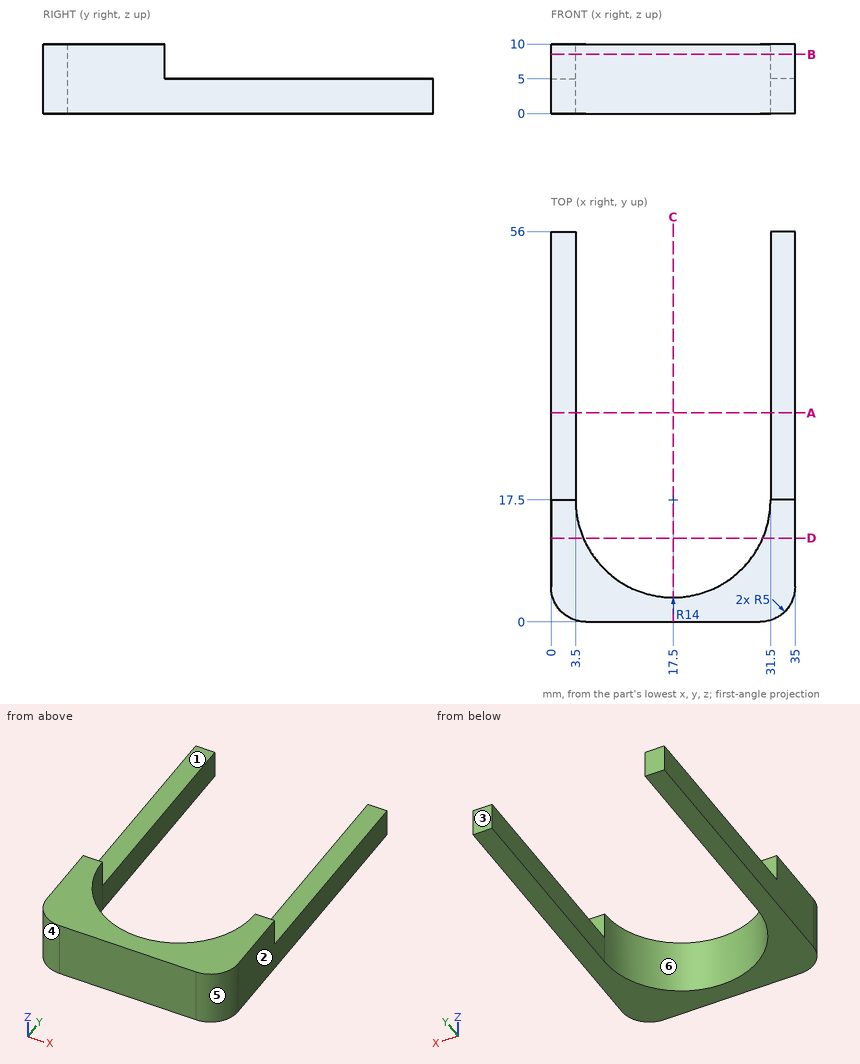
Geometry: see drawing. Coordinates: mm, zero at the bounding-box minimum. A direction names the side the tool comes from. Give positions to 0.01 mm unless a question says otherwise; leave off trailing zeros. Order: outer loops, then holes, each group sorted by start corner. A loop starts at its lowest first (then second) coordinate and runs counter-clockwise, first axis right, second up. Notation, with made-up numbers: (82.25, 44) - (123.25, 44) arc R22 ccw to (123.25, 56) - close; hole circle Ø11 at (12, 34.5). An arc over 180 degrees is marked (long way). One line per item, written item: value.
1. Cut plane B-B, the plane z = 8.5. Output: boundary loops of the cut face in (x, y).
Determined:
outline: (0, 5) arc R5 ccw to (5, 0) - (30, 0) arc R5 ccw to (35, 5) - (35, 17.5) - (31.5, 17.5) arc R14 cw to (3.5, 17.5) - (0, 17.5) - close
2. Line query: probe 1 along X at (y, z) = (20, 3); probe 2 along Z at (x, y) = (33.5, 23); probe 3 along X at (y, z) = (6.5, 1.75). Output: solid intervals per line, ascending.
Determined:
probe 1: 0 to 3.5, 31.5 to 35
probe 2: 0 to 5
probe 3: 0 to 8.84, 26.16 to 35
3. Cut plane C-C, the plane x = 17.5. Output: boundary loops of the cut face in (y, z).
Determined:
outline: (0, 0) - (3.5, 0) - (3.5, 10) - (0, 10) - close
4. Pin query (flat end, axial travel): pin 1 Ø1.5 at (y, z) = (41, 3.5) entering from -X; pin 2 Ø6 at (x, z) = (10.5, 8.5) entering from +Y; pin 3 Ø1.8 at (x, z) = (2.5, 7) entering from +Y; pin 4 Ø1 at (x, y) = (33, 28.5) entering from +Z. Return the tip coordinate at first contact, or that it passes through.
Determined:
pin 1: x = 0
pin 2: y = 7.7
pin 3: y = 17.5
pin 4: z = 5
5. Cut plane A-A, the plane y = 30. Output: boundary loops of the cut face in (x, z).
Determined:
outline: (0, 0) - (3.5, 0) - (3.5, 5) - (0, 5) - close; (31.5, 0) - (35, 0) - (35, 5) - (31.5, 5) - close
6. Draft query along X for the marked faces 3, 4, 5 and 6. Return one class per face: released by +X, released by -X, zero draft, split by the parting line, or undercut.
Determined:
face 3: zero draft
face 4: released by -X
face 5: released by +X
face 6: undercut
7. Cut plane D-D, the plane y = 12. Output: boundary loops of the cut face in (x, z), and give its area (3 significant figures).
Determined:
outline: (0, 0) - (4.63, 0) - (4.63, 10) - (0, 10) - close; (30.37, 0) - (35, 0) - (35, 10) - (30.37, 10) - close
area: 92.5 mm2
8. Reachability of the marked faces 1 and 2 from +Z, -Z, +X, -X, +Y, -Y: full face, straight path, thin tool, end or side. Return the list, or none.
Determined:
face 1: +Z, +X, -X, +Y
face 2: +Z, -Z, +X, +Y, -Y
